The listing builds one solid part. Answer for the finished solid, in the listing's coordinates (mm). A direction names the side the tool comes from. Round coordinates to 2 decimals unless told otherwise and drop trailing zeros. Order: outer loops, then holes, each group sorted by start corner. A loop starts at its lowest first (then second) coordinate and runs counter-clockwise, first axis right, second up. Notation, with made-up numbers: (40.25, 56.5) - (98.25, 56.5) arc R27 ccw to (98.25, 77.5) - close; hole circle Ø8 at (-30.75, 63). An arc over 180 degrees is marked (long way). One line per item, written item: value. Start each with the question number.
1. For a pull along Z with two mould halves and no side action, classify faces 1 (the cylindrical face through (6.434, 64.352, -11.803)), 2 (the flat face through (0, 36, -14)), 3 (the flat face through (-6, 0.8, 2)) as released by +Z, released by -Z, zero draft, split by the parting line, or undercut.
2. Section B-B, the plane y = 38 is taken. Give the vertices of the cut face in (x, z), then the cut area to 3 significant figures.
3. Section C-C, the plane z = 0 is taken. Count the separate pieces of the cut face and the enclosed holes in it, then the cut area to 3 significant figures.
4. Section A-A, the plane z = 8 is taken. Give the vertices of the cut face in (x, y), then the cut area to 3 significant figures.
5. A tool of negligible diameter and unlimited length cuts with its end or side. For faces 4 (the flat face through (-11, 66, 1)), 5 (the flat face through (0, 8.2, 8)), 6 (the flat face through (-10.5, 50, 0)), 7 (the cylindrical face through (-2.91, 0.41, -8.92)), from which of +Z, -Z, +X, -X, +Y, -Y can it reach the whole face along a straight path? Write none if from no direction.
6. Straight lines are drawn through the part: line 1 (X direction, y = 65.5, z = -7.25); line 2 (X direction, y = 3, z = 0); line 3 (Z direction, x = -1, y = 29). For each, find the intervals that lie inside material, in ascending order.
7. Flat-ended cylindrical pins translate along their axes: P1, Ø10, axis at x = -6, y = 64, coming from the +Z side; P2, Ø4.5, axis at x = 0, z = 8, coming from the +Y side; P3, Ø3, axis at x = -5, y = 62.5, coming from the +Z side; P4, Ø2, axis at x = 8, z = -4.5, coming from the +Y side. Find the tip coordinate at first contact, or state that the pin passes through.
from build123d import *

# Parameters (mm, degrees)
SKIZZE1_W                        = 28
SKIZZE1_H                        = 28
AUFSATZ_LINEAR_AUSTRAGEN1_DEPTH  = 72
SKIZZE2_W                        = 12.2
SKIZZE2_H                        = 10.2
SCHNITT_LINEAR_AUSTRAGEN1_DEPTH  = 53
SKIZZE3_W                        = 21
SKIZZE3_H                        = 24
SCHNITT_LINEAR_AUSTRAGEN2_DEPTH  = 44
SKIZZE6_R                        = 1.25
SCHNITT_LINEAR_AUSTRAGEN4_DEPTH  = 6
SCHNITT_LINEAR_AUSTRAGEN13_DEPTH = 2
SKIZZE7_W                        = 23.2
SKIZZE7_H                        = 26.2
SCHNITT_LINEAR_AUSTRAGEN5_DEPTH  = 1
SCHNITT_LINEAR_AUSTRAGEN14_DEPTH = 1.1
SKIZZE13_R                       = 3
SCHNITT_LINEAR_AUSTRAGEN11_DEPTH = 3
SCHNITT_LINEAR_START             = -3
SKIZZE11_R                       = 3
SCHNITT_LINEAR_AUSTRAGEN9_DEPTH  = 3
SKIZZE12_R                       = 1.625
SCHNITT_LINEAR_AUSTRAGEN10_DEPTH = 0.5
SKIZZE14_R                       = 1.65
SCHNITT_LINEAR_AUSTRAGEN12_DEPTH = 0.5
SKIZZE18_R                       = 2
AUFSATZ_LINEAR_AUSTRAGEN2_DEPTH  = 0.4
SKIZZE19_R                       = 0.75
SCHNITT_LINEAR_AUSTRAGEN15_DEPTH = 1.6
KREISMUSTER1_COUNT               = 4
VERRUNDUNG1_R                    = 1


with BuildPart() as part:
    # Skizze1 → Aufsatz-Linear austragen1 (new body)
    with BuildSketch(Plane(origin=(0, 0, 0), x_dir=(1, 0, 0), z_dir=(0, 1, 0))):
        Rectangle(SKIZZE1_W, SKIZZE1_H)
    extrude(amount=AUFSATZ_LINEAR_AUSTRAGEN1_DEPTH)

    # Skizze2 → Schnitt-Linear austragen1 (cut)
    with BuildSketch(Plane(origin=(0, 72, 0), x_dir=(1, 0, 0), z_dir=(0, 1, 0))):
        Rectangle(SKIZZE2_W, SKIZZE2_H)
    extrude(amount=-SCHNITT_LINEAR_AUSTRAGEN1_DEPTH, mode=Mode.SUBTRACT)

    # Skizze3 → Schnitt-Linear austragen2 (cut)
    with BuildSketch(Plane(origin=(0, 72, 0), x_dir=(1, 0, 0), z_dir=(0, 1, 0))):
        Rectangle(SKIZZE3_W, SKIZZE3_H)
    extrude(amount=-SCHNITT_LINEAR_AUSTRAGEN2_DEPTH, mode=Mode.SUBTRACT)

    # Skizze5 → Schnitt-Rotation1 (revolve, cut)
    with BuildSketch(Plane.XY, mode=Mode.PRIVATE) as schnitt_rotation1_sk:
        Polygon((-3, 0), (-3, 8), (-4.1, 8), (-4.1, 19), (0, 19), (0, 0), align=None)
    revolve(schnitt_rotation1_sk.sketch.rotate(Axis((0, 0, 0), (0, 1, 0)), 270), axis=Axis((0, 0, 0), (0, 1, 0)), mode=Mode.SUBTRACT)

    # Skizze6 → Schnitt-Linear austragen4 (cut)
    with BuildSketch(Plane(origin=(0, 28, 0), x_dir=(1, 0, 0), z_dir=(0, 1, 0))):
        with Locations(Location((7.9, 4.6, 0), (0, 0, 270))):
            Circle(SKIZZE6_R)
        with Locations(Location((-7.9, -4.6, 0), (0, 0, 270))):
            Circle(SKIZZE6_R)
    extrude(amount=-SCHNITT_LINEAR_AUSTRAGEN4_DEPTH, mode=Mode.SUBTRACT)

    # Skizze15 → Schnitt-Linear austragen13 (cut)
    with BuildSketch(Plane.XY.offset(14)):
        Polygon((10, 72), (-10, 72), (-8, 60), (8, 60), align=None)
    extrude(amount=-SCHNITT_LINEAR_AUSTRAGEN13_DEPTH, mode=Mode.SUBTRACT)

    # Skizze7 → Schnitt-Linear austragen5 (cut)
    with BuildSketch(Plane(origin=(0, 72, 0), x_dir=(1, 0, 0), z_dir=(0, 1, 0))):
        Rectangle(SKIZZE7_W, SKIZZE7_H)
    extrude(amount=-SCHNITT_LINEAR_AUSTRAGEN5_DEPTH, mode=Mode.SUBTRACT)

    # Skizze17 → Schnitt-Linear austragen14 (cut)
    with BuildSketch(Plane(origin=(0, 0, 12), x_dir=(-1, 0, 0), z_dir=(0, 0, -1))):
        Polygon((-8, 58.9), (-10.016666667, 71), (-9.833333333, 71), (-8, 60), (8, 60), (9.833333333, 71), (10.016666667, 71), (8, 58.9), align=None)
    extrude(amount=-SCHNITT_LINEAR_AUSTRAGEN14_DEPTH, mode=Mode.SUBTRACT)

    # Skizze13 → Schnitt-Linear austragen11 (cut)
    with BuildSketch(Plane.ZY.offset(14)):
        with Locations((0, 67.5)):
            Circle(SKIZZE13_R)
    extrude(amount=-SCHNITT_LINEAR_AUSTRAGEN11_DEPTH, mode=Mode.SUBTRACT)

    # Skizze11 → Schnitt-Linear austragen9 (cut)
    with BuildSketch(Plane(origin=(14, 0, 0), x_dir=(0, 0, -1), z_dir=(1, 0, 0)).offset(SCHNITT_LINEAR_START)):
        with Locations(Location((0, 67.5, 0), (0, 0, 180))):
            Circle(SKIZZE11_R)
    extrude(amount=SCHNITT_LINEAR_AUSTRAGEN9_DEPTH, mode=Mode.SUBTRACT)

    # Skizze12 → Schnitt-Linear austragen10 (cut)
    with BuildSketch(Plane(origin=(11, 0, 0), x_dir=(0, 0, -1), z_dir=(1, 0, 0))):
        with Locations((0, 67.5)):
            Circle(SKIZZE12_R)
    extrude(amount=-SCHNITT_LINEAR_AUSTRAGEN10_DEPTH, mode=Mode.SUBTRACT)

    # Skizze14 → Schnitt-Linear austragen12 (cut)
    with BuildSketch(Plane.ZY.offset(11)):
        with Locations((0, 67.5)):
            Circle(SKIZZE14_R)
    extrude(amount=-SCHNITT_LINEAR_AUSTRAGEN12_DEPTH, mode=Mode.SUBTRACT)

    # Skizze18 → Aufsatz-Linear austragen2 (add)
    with BuildSketch(Plane.XY.offset(-12)):
        with Locations(Location((-6, 62.4, 0), (0, 0, 180))):
            Circle(SKIZZE18_R)
        with Locations(Location((6, 62.4, 0), (0, 0, 180))):
            Circle(SKIZZE18_R)
    extrude(amount=AUFSATZ_LINEAR_AUSTRAGEN2_DEPTH)

    # Skizze19 → Schnitt-Linear austragen15 (cut)
    with BuildSketch(Plane.XY.offset(-11.6)):
        with Locations((-6, 62.4)):
            Circle(SKIZZE19_R)
        with Locations((6, 62.4)):
            Circle(SKIZZE19_R)
    extrude(amount=-SCHNITT_LINEAR_AUSTRAGEN15_DEPTH, mode=Mode.SUBTRACT)

    # Skizze20 → Schnitt-Rotation2 (revolve, cut)
    with BuildSketch(Plane.XY, mode=Mode.PRIVATE) as schnitt_rotation2_sk:
        Polygon((-4.95, 0), (-4.95, 0.8), (-5.45, 0.8), (-5.45, 7), (-4.95, 7), (-4.95, 8.2), (-8, 8.2), (-8, 0), align=None)
    schnitt_rotation2 = revolve(schnitt_rotation2_sk.sketch.rotate(Axis((-8, 8.2, 0), (0, -1, 0)), 90), axis=Axis((-8, 8.2, 0), (0, -1, 0)), mode=Mode.SUBTRACT)

    # Kreismuster1: Schnitt-Rotation2 ×4 about axis
    kreismuster1_axis = Axis((0, 0, 0), (0, 1, 0))
    for i in range(1, KREISMUSTER1_COUNT):
        add(schnitt_rotation2.rotate(kreismuster1_axis, i * 360 / KREISMUSTER1_COUNT), mode=Mode.SUBTRACT)

    # Verrundung1
    # the kernel refuses this fillet: 1 mm, written as the material it takes off along each edge
    with BuildSketch(Plane(origin=(-13, 1, -13), x_dir=(-1, 0, 0), z_dir=(0, 0, -1))) as verrundung1_piece_1_section:
        Polygon((0, 0), (VERRUNDUNG1_R, 0), (VERRUNDUNG1_R, -VERRUNDUNG1_R), (0, -VERRUNDUNG1_R), align=None)
    verrundung1_piece_1 = extrude(amount=VERRUNDUNG1_R, mode=Mode.PRIVATE)
    verrundung1_piece_1 = verrundung1_piece_1 - Plane(origin=(-13, 1, -13), x_dir=(0.7071067811865475, 0.7071067811865475, 0), z_dir=(0, 0, -1)) * Sphere(VERRUNDUNG1_R, mode=Mode.PRIVATE)
    add(verrundung1_piece_1, mode=Mode.SUBTRACT)
    with BuildSketch(Plane(origin=(-13, 1, 13), x_dir=(0, -1, 0), z_dir=(-1, 0, 0))) as verrundung1_piece_2_section:
        Polygon((0, 0), (VERRUNDUNG1_R, 0), (VERRUNDUNG1_R, VERRUNDUNG1_R), (0, VERRUNDUNG1_R), align=None)
    verrundung1_piece_2 = extrude(amount=VERRUNDUNG1_R, mode=Mode.PRIVATE)
    verrundung1_piece_2 = verrundung1_piece_2 - Plane(origin=(-13, 1, 13), x_dir=(0, 0.7071067811865475, -0.7071067811865475), z_dir=(-1, 0, 0)) * Sphere(VERRUNDUNG1_R, mode=Mode.PRIVATE)
    add(verrundung1_piece_2, mode=Mode.SUBTRACT)
    with BuildSketch(Plane(origin=(13, 1, 13), x_dir=(0, -1, 0), z_dir=(1, 0, 0))) as verrundung1_piece_3_section:
        Polygon((0, 0), (VERRUNDUNG1_R, 0), (VERRUNDUNG1_R, -VERRUNDUNG1_R), (0, -VERRUNDUNG1_R), align=None)
    verrundung1_piece_3 = extrude(amount=VERRUNDUNG1_R, mode=Mode.PRIVATE)
    verrundung1_piece_3 = verrundung1_piece_3 - Plane(origin=(13, 1, 13), x_dir=(0, 0.7071067811865475, -0.7071067811865475), z_dir=(1, 0, 0)) * Sphere(VERRUNDUNG1_R, mode=Mode.PRIVATE)
    add(verrundung1_piece_3, mode=Mode.SUBTRACT)
    with BuildSketch(Plane(origin=(13, 1, -13), x_dir=(1, 0, 0), z_dir=(0, 0, -1))) as verrundung1_piece_4_section:
        Polygon((0, 0), (VERRUNDUNG1_R, 0), (VERRUNDUNG1_R, VERRUNDUNG1_R), (0, VERRUNDUNG1_R), align=None)
    verrundung1_piece_4 = extrude(amount=VERRUNDUNG1_R, mode=Mode.PRIVATE)
    verrundung1_piece_4 = verrundung1_piece_4 - Plane(origin=(13, 1, -13), x_dir=(-0.7071067811865475, 0.7071067811865475, 0), z_dir=(0, 0, -1)) * Sphere(VERRUNDUNG1_R, mode=Mode.PRIVATE)
    add(verrundung1_piece_4, mode=Mode.SUBTRACT)
    with BuildSketch(Plane(origin=(13, 71, 13), x_dir=(0, 1, 0), z_dir=(1, 0, 0))) as verrundung1_piece_5_section:
        Polygon((0, 0), (VERRUNDUNG1_R, 0), (VERRUNDUNG1_R, VERRUNDUNG1_R), (0, VERRUNDUNG1_R), align=None)
    verrundung1_piece_5 = extrude(amount=VERRUNDUNG1_R, mode=Mode.PRIVATE)
    verrundung1_piece_5 = verrundung1_piece_5 - Plane(origin=(13, 71, 13), x_dir=(0, -0.7071067811865475, -0.7071067811865475), z_dir=(1, 0, 0)) * Sphere(VERRUNDUNG1_R, mode=Mode.PRIVATE)
    add(verrundung1_piece_5, mode=Mode.SUBTRACT)
    with BuildSketch(Plane(origin=(13, 71, -13), x_dir=(1, 0, 0), z_dir=(0, 0, -1))) as verrundung1_piece_6_section:
        Polygon((0, 0), (VERRUNDUNG1_R, 0), (VERRUNDUNG1_R, -VERRUNDUNG1_R), (0, -VERRUNDUNG1_R), align=None)
    verrundung1_piece_6 = extrude(amount=VERRUNDUNG1_R, mode=Mode.PRIVATE)
    verrundung1_piece_6 = verrundung1_piece_6 - Plane(origin=(13, 71, -13), x_dir=(-0.7071067811865475, -0.7071067811865475, 0), z_dir=(0, 0, -1)) * Sphere(VERRUNDUNG1_R, mode=Mode.PRIVATE)
    add(verrundung1_piece_6, mode=Mode.SUBTRACT)
    with BuildSketch(Plane(origin=(-13, 71, -13), x_dir=(-1, 0, 0), z_dir=(0, 0, -1))) as verrundung1_piece_7_section:
        Polygon((0, 0), (VERRUNDUNG1_R, 0), (VERRUNDUNG1_R, VERRUNDUNG1_R), (0, VERRUNDUNG1_R), align=None)
    verrundung1_piece_7 = extrude(amount=VERRUNDUNG1_R, mode=Mode.PRIVATE)
    verrundung1_piece_7 = verrundung1_piece_7 - Plane(origin=(-13, 71, -13), x_dir=(0.7071067811865475, -0.7071067811865475, 0), z_dir=(0, 0, -1)) * Sphere(VERRUNDUNG1_R, mode=Mode.PRIVATE)
    add(verrundung1_piece_7, mode=Mode.SUBTRACT)
    with BuildSketch(Plane(origin=(-13, 71, 13), x_dir=(0, 1, 0), z_dir=(-1, 0, 0))) as verrundung1_piece_8_section:
        Polygon((0, 0), (VERRUNDUNG1_R, 0), (VERRUNDUNG1_R, -VERRUNDUNG1_R), (0, -VERRUNDUNG1_R), align=None)
    verrundung1_piece_8 = extrude(amount=VERRUNDUNG1_R, mode=Mode.PRIVATE)
    verrundung1_piece_8 = verrundung1_piece_8 - Plane(origin=(-13, 71, 13), x_dir=(0, -0.7071067811865475, -0.7071067811865475), z_dir=(-1, 0, 0)) * Sphere(VERRUNDUNG1_R, mode=Mode.PRIVATE)
    add(verrundung1_piece_8, mode=Mode.SUBTRACT)
    with BuildSketch(Plane(origin=(-14, 0, -13), x_dir=(0, 1, 0), z_dir=(0, 0, 1)), Plane(origin=(14, 0, 13), x_dir=(0, 1, 0), z_dir=(0, 0, -1)), Plane(origin=(13, 0, -14), x_dir=(0, 1, 0), z_dir=(-1, 0, 0))) as verrundung1_piece_9:
        with BuildLine():
            CenterArc((VERRUNDUNG1_R, -VERRUNDUNG1_R), VERRUNDUNG1_R, 90, 90)
            Line((0, -VERRUNDUNG1_R), (0, 0))
            Line((0, 0), (VERRUNDUNG1_R, 0))
        make_face()
    extrude(amount=26, mode=Mode.SUBTRACT)
    with BuildSketch(Plane(origin=(-13, 0, 14), x_dir=(0, 0, -1), z_dir=(1, 0, 0)), Plane(origin=(13, 72, -14), x_dir=(0, -1, 0), z_dir=(-1, 0, 0)), Plane(origin=(14, 72, 13), x_dir=(0, -1, 0), z_dir=(0, 0, -1)), Plane(origin=(-14, 72, -13), x_dir=(0, -1, 0), z_dir=(0, 0, 1))) as verrundung1_piece_10:
        with BuildLine():
            CenterArc((VERRUNDUNG1_R, VERRUNDUNG1_R), VERRUNDUNG1_R, 180, 90)
            Line((0, VERRUNDUNG1_R), (0, 0))
            Line((0, 0), (VERRUNDUNG1_R, 0))
        make_face()
    extrude(amount=26, mode=Mode.SUBTRACT)
    with BuildSketch(Plane(origin=(14, 1, 14), x_dir=(0, 0, -1), z_dir=(0, 1, 0)), Plane(origin=(14, 1, -14), x_dir=(-1, 0, 0), z_dir=(0, 1, 0))) as verrundung1_piece_11:
        with BuildLine():
            CenterArc((VERRUNDUNG1_R, VERRUNDUNG1_R), VERRUNDUNG1_R, 180, 90)
            Line((0, VERRUNDUNG1_R), (0, 0))
            Line((0, 0), (VERRUNDUNG1_R, 0))
        make_face()
    extrude(amount=70, mode=Mode.SUBTRACT)
    with BuildSketch(Plane(origin=(-14, 1, -14), x_dir=(1, 0, 0), z_dir=(0, 1, 0)), Plane(origin=(-14, 1, 14), x_dir=(0, 0, -1), z_dir=(0, 1, 0))) as verrundung1_piece_12:
        with BuildLine():
            CenterArc((VERRUNDUNG1_R, -VERRUNDUNG1_R), VERRUNDUNG1_R, 90, 90)
            Line((0, -VERRUNDUNG1_R), (0, 0))
            Line((0, 0), (VERRUNDUNG1_R, 0))
        make_face()
    extrude(amount=70, mode=Mode.SUBTRACT)
    with BuildSketch(Plane(origin=(7.5, 72, 14), x_dir=(0, 0, -1), z_dir=(1, 0, 0)), Plane(origin=(-13, 72, 14), x_dir=(0, 0, -1), z_dir=(1, 0, 0))) as verrundung1_piece_13:
        with BuildLine():
            CenterArc((VERRUNDUNG1_R, -VERRUNDUNG1_R), VERRUNDUNG1_R, 90, 90)
            Line((0, -VERRUNDUNG1_R), (0, 0))
            Line((0, 0), (VERRUNDUNG1_R, 0))
        make_face()
    extrude(amount=5.5, mode=Mode.SUBTRACT)


solid = part.part
Answer list:
1. face 1: zero draft
1. face 2: released by -Z
1. face 3: undercut
2. outline: (-14, -13) arc R1 ccw to (-13, -14) - (13, -14) arc R1 ccw to (14, -13) - (14, 13) arc R1 ccw to (13, 14) - (-13, 14) arc R1 ccw to (-14, 13) - close; hole (-10.5, -12) - (10.5, -12) - (10.5, 12) - (-10.5, 12) - close
2. area: 279 mm²
3. separate pieces: 4
3. enclosed holes: 0
3. area: 714 mm²
4. outline: (-14, 1) arc R1 ccw to (-13, 0) - (-3.05, 0) - (-3.05, 0.8) - (-2.55, 0.8) - (-2.55, 7) - (-3.05, 7) - (-3.05, 8.2) - (3.05, 8.2) - (3.05, 7) - (2.55, 7) - (2.55, 0.8) - (3.05, 0.8) - (3.05, 0) - (13, 0) arc R1 ccw to (14, 1) - (14, 71) arc R1 ccw to (13, 72) - (11.6, 72) - (11.6, 71) - (10.5, 71) - (10.5, 28) - (-10.5, 28) - (-10.5, 71) - (-11.6, 71) - (-11.6, 72) - (-13, 72) arc R1 ccw to (-14, 71) - close
4. area: 1,050 mm²
5. face 4: -X
5. face 5: none
5. face 6: +Y
5. face 7: -Y
6. line 1: x = -14 to -10.5, 10.5 to 14
6. line 2: x = -14 to -10.55, -5.45 to -3, 3 to 5.45, 10.55 to 14
6. line 3: z = -14 to -12, 12 to 14
7. P1: stops at z = 14
7. P2: stops at y = 28
7. P3: stops at z = -11.6
7. P4: stops at y = 22
